Design review of the part built by this model. Coordinates are the model's own, in mm. A direction names the side the tool comes from. Round coordinates to 2 decimals unless told otherwise and drop trailing zeros. Order: outer loops, then holes, each group sorted by start corner. A loop starts at its lowest first (then second) coordinate and runs counter-clockwise, first axis right, second up. Notation, with made-up numbers: (77, 0) - (114, 0) arc R18 cw to (114, 28) - close; hole circle Ø11 at (-12.5, -19). An arc over 180 degrees is marked (long way). Answer as a JSON object with one key per item and string values. Group by question number.
from build123d import *

# Parameters (mm, degrees)
SKETCH1_R           = 25
BOSS_EXTRUDE1_DEPTH = 30
SKETCH2_W           = 50
SKETCH2_H           = 50.327363666
BOSS_EXTRUDE2_DEPTH = 40
FILLET1_R           = 10
SKETCH3_R           = 15
CUT_EXTRUDE1_DEPTH  = 10


with BuildPart() as part:
    # Sketch1 → Boss-Extrude1 (new body)
    with BuildSketch(Plane(origin=(0, 0, 0), x_dir=(0, 0, -1), z_dir=(1, 0, 0))):
        Circle(SKETCH1_R)
    extrude(amount=BOSS_EXTRUDE1_DEPTH)

    # Sketch2 → Boss-Extrude2 (add)
    with BuildSketch(Plane(origin=(30, 0, 0), x_dir=(0, 0, -1), z_dir=(1, 0, 0))):
        Rectangle(SKETCH2_W, SKETCH2_H)
    extrude(amount=BOSS_EXTRUDE2_DEPTH)

    # Fillet1
    fillet1_edges = [part.edges().sort_by_distance(p)[0] for p in [
        (70, 25.163681833, 0),
    ]]
    fillet(fillet1_edges, radius=FILLET1_R)

    # Sketch3 → Cut-Extrude1 (cut)
    with BuildSketch(Plane.XZ.offset(25.163681833)):
        with Locations(Location((50, 0, 0), (0, 0, 270))):
            Circle(SKETCH3_R)
    extrude(amount=-CUT_EXTRUDE1_DEPTH, mode=Mode.SUBTRACT)


solid = part.part
1. Take a section at B-B, the plane z = 0. Give the boundary of the cut face in (x, y).
2. Take a section at D-D, the plane z = 17.5. Give the boundary of the cut face in (x, y).
3. To check wall thickness, follow line 1 (X direction, y = -22, z = 0); line 2 (X direction, y = -19, z = 22.5); line 3 (Y direction, x = 57, z = 8.5). State the ranges of each line that lie inside material, in increasing order. Write a range as from..to.
4. Clearance check with flat-ended pins moving along their axes: P1, Ø12.5, axis at y = 8, z = -7, coming from the -X side; P2, Ø5, axis at y = 18.5, z = -12, coming from the +X side; P3, Ø18, axis at x = 50, z = 0, coming from the -Y side; P4, Ø3, axis at x = 8, y = 15.5, coming from the +Z side. State where each tip first meets the part, or that it passes through.
5. Tool access review of faces 4 (the flat face through (30, -25, -5)), 5 (the flat face through (50, 0, 25)), 6 (the cylindrical face through (64.872, -20.234, 1.953)): name each direction out of +Z, -Z, +X, -X, +Y, -Y from which nothing blocks a thin tool from reaching the whole face with its end or side.
6. Mouldability with a two-part tool opening along Z and no side actions: class faces 1 (the flat face through (50, -15.164, 0)), 2 (the cylindrical face through (14.79, 7.509, -23.846)), 3 (the flat face through (30, 25, -4)) as pulls with the +Z half, pulls with the -Z half, needs draft (parallel to the pull), parting line crosses it, or undercut.
7. Take a section at A-A, the plane x = 50. Give the boundary of the cut face in (y, z), then the cut area to 3 significant figures.
8. Take a section at C-C, the plane y = 13. Give the boundary of the cut face in (x, z), then the cut area to 3 significant figures.
Response values:
{
 "1": {"outline": "(0, -25) - (30, -25) - (30, -25.16) - (35, -25.16) - (35, -15.16) - (65, -15.16) - (65, -25.16) - (70, -25.16) - (70, 15.16) arc R10 ccw to (60, 25.16) - (30, 25.16) - (30, 25) - (0, 25) - close"},
 "2": {"outline": "(0, -17.85) - (30, -17.85) - (30, -25.16) - (70, -25.16) - (70, 15.16) arc R10 ccw to (60, 25.16) - (30, 25.16) - (30, 17.85) - (0, 17.85) - close"},
 "3": {"line 1": "0..35, 65..70", "line 2": "30..70", "line 3": "-15.16..25.16"},
 "4": {"P1": "x = 0", "P2": "x = 69.96", "P3": "y = -15.16", "P4": "z = 20.71"},
 "5": {"face 4": "-X, -Y", "face 5": "+Z, +X, -X, +Y, -Y", "face 6": "-Y"},
 "6": {"face 1": "undercut", "face 2": "parting line crosses it", "face 3": "needs draft"},
 "7": {"outline": "(-25.16, -25) - (25.16, -25) - (25.16, 25) - (-25.16, 25) - (-25.16, 15) - (-15.16, 15) - (-15.16, -15) - (-25.16, -15) - close", "area": "2,220 mm2"},
 "8": {"outline": "(0, -21.35) - (30, -21.35) - (30, -25) - (70, -25) - (70, 25) - (30, 25) - (30, 21.35) - (0, 21.35) - close", "area": "3,280 mm2"}
}
